Source: CAD feature listing. Evaluate the final solid. Frame: model axes, mm. Round coordinates to 2 decimals unless told otherwise and drop trailing zeros. Loops run counter-clockwise (first coordinate to the right, second up) from the corner with the lowest first, then second, coordinate; pieces in that order, holes last. Notation, with made-up numbers: (19.25, -23.75) -> (73.25, -23.75) arc R21 cw to (73.25, -8.75) -> close; hole circle Ø5 at (69.25, 2.25). An arc over 180 degrees is marked (long way). Write item = value, one per line.
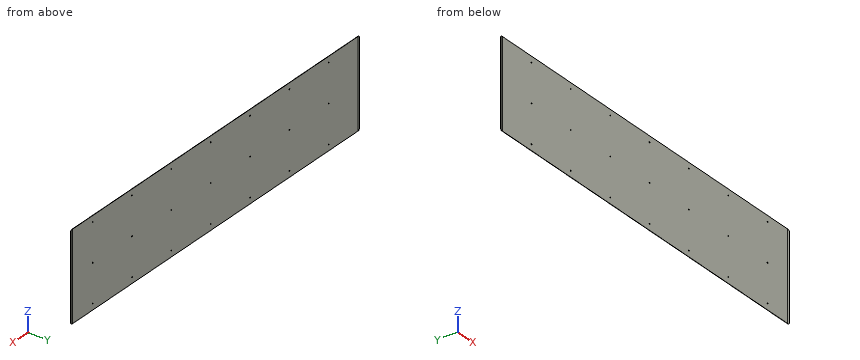
from build123d import *

# Parameters (mm, degrees)
ESTRUSIONE_ESTRUSIONE1_DEPTH = 254.5
RACCORDO1_R                  = 10
SCHIZZO2_R                   = 3
TAGLIO_ESTRUSIONE1_DEPTH     = 2
RIPETIZIONE_A_L1_COUNT       = 4
RIPETIZIONE_A_L1_PITCH       = 300
RIPETIZIONE_A_L1_COL_COUNT   = 4
RIPETIZIONE_A_L1_COL_PITCH   = 300


with BuildPart() as part:
    # Schizzo1 → Estrusione-Estrusione1 (new, symmetric)
    with BuildSketch(Plane.XY):
        with BuildLine():
            Line((-1089.232382107, 0.706239028), (-1100, -0.235805471))
            Line((-1100, -0.235805471), (-1099.860182927, -1.833921932))
            Line((-1099.860182927, -1.833921932), (-1087.90584655, -0.788053019))
            ThreePointArc((-1087.90584655, -0.788053019), (-1087.470482996, -0.759517784), (-1087.034289122, -0.75))
            Line((-1087.034289122, -0.75), (1087.034289122, -0.75))
            ThreePointArc((1087.034289122, -0.75), (1087.470482996, -0.759517784), (1087.90584655, -0.788053019))
            Line((1087.90584655, -0.788053019), (1099.860182927, -1.833921932))
            Line((1099.860182927, -1.833921932), (1100, -0.235805471))
            Line((1100, -0.235805471), (1089.232382107, 0.706239028))
            ThreePointArc((1089.232382107, 0.706239028), (1088.73171402, 0.739054548), (1088.230091065, 0.75))
            Line((1088.230091065, 0.75), (-1088.230091065, 0.75))
            ThreePointArc((-1088.230091065, 0.75), (-1088.73171402, 0.739054548), (-1089.232382107, 0.706239028))
        make_face()
    extrude(amount=ESTRUSIONE_ESTRUSIONE1_DEPTH, both=True)

    # Raccordo1
    raccordo1_edges = [part.edges().sort_by_distance(p)[0] for p in [
        (1099.930091463, -1.034863701, -254.5),
        (-1099.930091463, -1.034863701, -254.5),
        (1099.930091463, -1.034863701, 254.5),
        (-1099.930091463, -1.034863701, 254.5),
    ]]
    fillet(raccordo1_edges, radius=RACCORDO1_R)

    # Schizzo2 → Taglio-Estrusione1 (cut)
    with BuildSketch(Plane(origin=(0, 0.75, 0), x_dir=(1, 0, 0), z_dir=(0, 1, 0))):
        with Locations(Location((35, -220, 0), (0, 0, 180))):
            Circle(SCHIZZO2_R)
        with Locations(Location((35, 220, 0), (0, 0, 180))):
            Circle(SCHIZZO2_R)
        with Locations(Location((35, 0, 0), (0, 0, 180))):
            Circle(SCHIZZO2_R)
    taglio_estrusione1 = extrude(amount=-TAGLIO_ESTRUSIONE1_DEPTH, mode=Mode.SUBTRACT)

    # Ripetizione a L1: Taglio-Estrusione1 ×4
    with Locations(*[(i * RIPETIZIONE_A_L1_PITCH, 0, 0) for i in range(1, RIPETIZIONE_A_L1_COUNT)]):
        add(taglio_estrusione1, mode=Mode.SUBTRACT)

    # Ripetizione a L1 col: Taglio-Estrusione1 ×4
    with Locations(*[(-i * RIPETIZIONE_A_L1_COL_PITCH, 0, 0) for i in range(1, RIPETIZIONE_A_L1_COL_COUNT)]):
        add(taglio_estrusione1, mode=Mode.SUBTRACT)


solid = part.part
1. Section query B-B (x = 553.5). Return the cut outline in (y, z), then the cut area to 4 significant figures.
Evaluation:
outline = (-0.75, -254.5) -> (0.75, -254.5) -> (0.75, 254.5) -> (-0.75, 254.5) -> close
area = 763.5 mm²
2. Section query A-A (z = -108.5). Return the cut outline in (x, y).
Evaluation:
outline = (-1100, -0.24) -> (-1099.86, -1.83) -> (-1087.91, -0.79) arc R10 cw to (-1087.03, -0.75) -> (1087.03, -0.75) arc R10 cw to (1087.91, -0.79) -> (1099.86, -1.83) -> (1100, -0.24) -> (1089.23, 0.71) arc R11.5 ccw to (1088.23, 0.75) -> (-1088.23, 0.75) arc R11.5 ccw to (-1089.23, 0.71) -> close
3. Line query: probe 1 along Z at (x, y) = (34, -0.7); probe 2 along Z at (x, y) = (-865, 0.2); probe 3 along Y at (x, z) = (965, -46.5). Output: solid intervals per line, ascending. Write a range as from..to.
Evaluation:
probe_1 = -254.5..-222.83, -217.17..-2.83, 2.83..217.17, 222.83..254.5
probe_2 = -254.5..-223, -217..-3, 3..217, 223..254.5
probe_3 = -0.75..0.75
4. Contact query for flat-ended pins moving along their axis: pin 1 Ø8 at (x, z) = (-865, -220) entering from +Y; pin 2 Ø7 at (x, z) = (-265, -220) entering from -Y. Output: stop coordinate, or through.
Evaluation:
pin_1 = 0.75
pin_2 = -0.75
